```python
from build123d import *
from build123d.topology import SkipClean

# Parameters (mm, degrees)
SKETCH1_W               = 69.342
SKETCH1_H               = 33.655
BOSS_EXTRUDE1_DEPTH     = 21.336
CUT_EXTRUDE2_DEPTH      = 53.820092408
CUT_EXTRUDE2_DEPTH_BACK = 53.820092408
FILLET1_R               = 2.54
SKETCH3_R               = 1.524
BOSS_EXTRUDE2_DEPTH     = 3.81
SKETCH5_R               = 1.524
SKETCH5_3_R             = 1.524


with BuildPart() as part:
    # Sketch1 → Boss-Extrude1 (new body)
    with BuildSketch(Plane(origin=(0, 0, 0), x_dir=(1, 0, 0), z_dir=(0, 1, 0))):
        Rectangle(SKETCH1_W, SKETCH1_H)
    extrude(amount=BOSS_EXTRUDE1_DEPTH)

    # Sketch2 → Cut-Extrude2 (cut, two sides: drawn at the far end of the back side and taken through both)
    with BuildSketch(Plane.XY.offset(16.8275).offset(-CUT_EXTRUDE2_DEPTH_BACK)):
        with BuildLine():
            Line((30.937128183, 158.024775042), (-32.322112251, 21.336))
            ThreePointArc((-32.322112251, 21.336), (-34.671, 10.668), (-32.322112251, 0))
            Line((-32.322112251, 0), (30.937128183, -136.688775042))
            Line((30.937128183, -136.688775042), (-270.297350074, -136.688775042))
            Line((-270.297350074, -136.688775042), (-270.297350074, 158.024775042))
            Line((-270.297350074, 158.024775042), (30.937128183, 158.024775042))
        make_face()
    extrude(amount=CUT_EXTRUDE2_DEPTH + CUT_EXTRUDE2_DEPTH_BACK, mode=Mode.SUBTRACT)

    # Fillet1
    fillet1_edges = [part.edges().sort_by_distance(p)[0] for p in [
        (34.671, 21.336, 0),
        (1.174443875, 21.336, -16.8275),
        (1.174443875, 0, 16.8275),
        (-32.322112251, 0, 0),
        (1.174443875, 21.336, 16.8275),
        (-32.322112251, 21.336, 0),
        (-34.671, 10.668, 16.8275),
        (-34.671, 10.668, -16.8275),
        (1.174443875, 0, -16.8275),
        (34.671, 0, 0),
        (34.671, 10.668, -16.8275),
        (34.671, 10.668, 16.8275),
    ]]
    fillet(fillet1_edges, radius=FILLET1_R)

    # Sketch3 → Boss-Extrude2 (add)
    with BuildSketch(Plane.ZY.offset(32.322112251)):
        with Locations(Location((-12.7635, 12.56538, 0), (0, 0, 180))):
            Circle(SKETCH3_R)
        with Locations(Location((-12.7635, 4.699, 0), (0, 0, 180))):
            Circle(SKETCH3_R)
    extrude(amount=BOSS_EXTRUDE2_DEPTH)

    # Sweep1: sweep along a path in Sketch4
    with SkipClean():  # the faces are left unmerged after this step: merging them gives an invalid solid
        with BuildLine(Plane.XY.offset(-12.7635)) as sweep1_path:
            Line((-36.132112251, 12.56538), (-48.832112251, 12.56538))
            Line((-48.832112251, 12.56538), (-112.332112251, 12.56538))
        # Sketch5 → Sweep1 (sweep)
        with BuildSketch(Plane.ZY.offset(36.132112251)):
            with Locations((-12.7635, 12.56538)):
                Circle(SKETCH5_R)
        sweep(path=sweep1_path.line)

    # Sweep2: sweep along a path in Sketch4<3>
    with SkipClean():  # the faces are left unmerged after this step: merging them gives an invalid solid
        with BuildLine(Plane.XY.offset(-12.7635)) as sweep2_path:
            ThreePointArc((-36.132112251, 4.699), (-39.516811705, 5.304169163), (-42.482112251, 7.04469))
            ThreePointArc((-42.482112251, 7.04469), (-45.447412797, 8.785210837), (-48.832112251, 9.39038))
            Line((-48.832112251, 9.39038), (-99.632112251, 9.39038))
            ThreePointArc((-99.632112251, 9.39038), (-103.016811705, 8.785210837), (-105.982112251, 7.04469))
            ThreePointArc((-105.982112251, 7.04469), (-108.947412797, 5.304169163), (-112.332112251, 4.699))
        # Sketch5<3> → Sweep2 (sweep)
        with BuildSketch(Plane.ZY.offset(36.132112251)):
            with Locations((-12.7635, 4.699)):
                Circle(SKETCH5_3_R)
        sweep(path=sweep2_path.line)


solid = part.part
```
Design review of the part built by this model. Coordinates are the model's own, in mm. A direction names the side the tool comes from. Give positions to 0.01 mm unless a question says otherwise; leave off trailing zeros. Loops run counter-clockwise (first coordinate to the right, second up) from the corner with the lowest first, then second, coordinate; pieces in that order, holes last. Notation, with made-up numbers: M 12.5,20.25 L 40.5,20.25 A10 ccw 40.5,27.25 Z; hole C 57.25,-9.5 d5. An arc over 180 degrees is marked long. Return JSON: item names as keys, results as strings. Group by question number.
Item 1: We need section B-B (x = -56.5). Give the boundary of the cut face in (y, z).
Item 2: We need section A-A (z = 9.5). Give the boundary of the cut face in (x, y).
Item 3: Tool access review of faces 4 (the cylindrical face through (-35.106, 3.188, -12.565)), 5 (the flat face through (-112.332, 13, -13)): name each direction out of +Z, -Z, +X, -X, +Y, -Y from which nothing blocks a thin tool from reaching the whole face with its end or side.
Item 4: Mouldability with a two-part tool opening along X and no side actions: class faces 1 (the cylindrical face through (33.95, 20.57, -0.2)), 2 (the cylindrical face through (-74.588, 10.675, -11.944)), 3 (the cylindrical face through (1.186, 20.572, 16.103)) as released by +X, released by -X, zero draft, split by the parting line, or undercut.
Item 5: Insertion check: pin 1 Ø12 at (x, y) = (-57, 16) entering from -Z; pin 2 Ø12 at (x, y) = (-83.5, 4) entering from +Z; pin 3 Ø3 at (y, z) = (14, 1.5) entering from -X. Each pin has a flat end and moves straight along its axis. Give the tip position at first contact, or say it passes through.
Item 6: For probe 1 along X at (y, z) = (10.5, -11); probe 2 along X at (y, z) = (14, 8); probe 3 along Y at (x, z) = (-4, 14.5), list the stretches that pass through material, from the lowest coordinate up.
Output:
{
 "1": {"outline": "C 9.39,-12.76 d3.05; C 12.57,-12.76 d3.05"},
 "2": {"outline": "M -33.01,1.64 A2.54 ccw -30.64,0 L 32.13,0 A2.54 ccw 34.67,2.54 L 34.67,18.8 A2.54 ccw 32.13,21.34 L -30.64,21.34 A2.54 ccw -33.01,19.7 A25.4 ccw Z"},
 "3": {"face 4": "none", "face 5": "+Z, -Z, -X, +Y, -Y"},
 "4": {"face 1": "released by +X", "face 2": "undercut", "face 3": "zero draft"},
 "5": {"pin 1": "stops at z = -14.29", "pin 2": "stops at z = -11.24", "pin 3": "stops at x = -34.6"},
 "6": {"probe 1": "x = -34.67 to 34.67", "probe 2": "x = -34.45 to 34.67", "probe 3": "y = 0.01 to 21.33"}
}
